Read the model definition and answer for the solid it produces. Units are mm, in the model's axes. A direction names the side the tool comes from. Round coordinates to 2 decimals unless told otherwise and drop trailing zeros. Order: outer loops, then holes, each group sorted by start corner. A loop starts at its lowest first (then second) coordinate and runs counter-clockwise, first axis right, second up. Notation, with made-up numbers: (19.25, 19.25) - (26.25, 19.25) arc R9 ccw to (26.25, 30.25) - close; hole circle Ø1 at (-19.75, 26). An arc over 180 degrees is marked (long way). Put each result on its own line as item: value. Start each with the question number.
Q1. Section A-A on y = 10.5 is taken. Give the vertices of the cut face in (x, z).
Q2. Find the intervals of material crossed by line 1 along Y through (x, z) = (78, 0.9); line 2 along X through (y, z) = (9, 0.65); line 3 along Y through (x, z) = (-83, 2.6), in increasing order. Write a range as from..to.
Q3. Which of the six approach directions +Z, -Z, +X, -X, +Y, -Y give full straight-line access (tool end or side, diameter ignored) to faces 4 (the face through (52.5, -21, 2)), 5 (the face through (-87, -20, 1)), 6 (the face through (0, 20, 1)), 7 (the face through (86, -20, 1))?
Q4. For a pull along X with two mould halves and no side action, classify faces 1 (the face through (89, -1, 1)), 2 (the face through (-90.5, -18, 1)), 3 (the face through (52.5, 22, 2)) as pulls with the +X half, pulls with the -X half, needs draft (parallel to the pull), parting line crosses it, or undercut.
Q5. Section C-C on y = -7 is taken. Give the vertices of the cut face in (x, z).
Q6. Each of these flat-tipped pins is pushed along its axis until it touches: pin 1 Ø0.9 at (x, z) = (-3.5, 2) entering from +Y; pin 2 Ø1.5 at (x, z) = (89, 1.5) entering from +Y; pin 3 Ø1.5 at (x, z) = (30.5, 1.5) entering from -Y. Where does it stop, or does it pass through?
Q7. Section B-B on x = 78 is taken. Give the vertices of the cut face in (y, z).
Q8. Section D-D on z = 2.05 is taken. State how many separate pieces and enclosed holes the cut face has, then the cut area to 3 significant figures.
Autodesk Inventor part; units mm, degrees
ref_plane "YZ Plane" through (0, 0, 0) normal (1, 0, 0) x (0, 1, 0)
ref_plane "XZ Plane" through (0, 0, 0) normal (0, 1, 0) x (-1, 0, 0)
ref_plane "XY Plane" through (0, 0, 0) normal (0, 0, 1) x (1, 0, 0)
sketch "Sketch1" plane through (0, 0, 0) normal (0, 0, 1) x (1, 0, 0)
  line L0 (-87.5, -20) -> (87.5, -20)
  line L1 (87.5, -20) -> (87.5, 20)
  line L2 (87.5, 20) -> (-87.5, 20)
  line L3 (-87.5, 20) -> (-87.5, -20)
  line L4 (-87.5, -20) -> (87.5, 20) construction
  line L5 (87.5, -20) -> (-87.5, 20) construction
  line L6 (-87.5, 14) -> (-90.5, 14)
  line L7 (-90.5, 14) -> (-90.5, -1)
  line L8 (-90.5, -1) -> (-87.5, -1)
  line L9 (-87.5, -1) -> (-87.5, 14)
  line L10 (-87.5, -20) -> (-90.5, -20)
  line L11 (-90.5, -20) -> (-90.5, -16)
  line L12 (-90.5, -16) -> (-87.5, -16)
  line L13 (-87.5, -16) -> (-87.5, -20)
  line L14 (0, 20) -> (0, -20) construction
  line L15 (87.5, 14) -> (90.5, 14)
  line L16 (90.5, 14) -> (90.5, -1)
  line L17 (90.5, -1) -> (87.5, -1)
  line L18 (87.5, -1) -> (87.5, 14)
  line L19 (87.5, -20) -> (90.5, -20)
  line L20 (90.5, -20) -> (90.5, -16)
  line L21 (90.5, -16) -> (87.5, -16)
  line L22 (87.5, -16) -> (87.5, -20)
  point P0 (0, 0)
  dimension "d0" = 175
  dimension "d1" = 40
  dimension "d2" = 3
  dimension "d3" = 15
  dimension "d4" = 6
  dimension "d5" = 3
  dimension "d6" = 15
extrude "Extrusion1" add sketch "Sketch1" along normal blind 3
sketch "Sketch2" plane through (0, 0, 3) normal (0, 0, 1) x (1, 0, 0)
  line L0 (-90.5, -20) -> (90.5, -20)
  line L1 (-82.5, -20) -> (-67.5, -20)
  line L2 (-67.5, -20) -> (-67.5, -23)
  line L3 (-67.5, -23) -> (-82.5, -23)
  line L4 (-82.5, -23) -> (-82.5, -20)
  line L5 (-52.5, -20) -> (-37.5, -20)
  line L6 (-37.5, -20) -> (-37.5, -23)
  line L7 (-37.5, -23) -> (-52.5, -23)
  line L8 (-52.5, -23) -> (-52.5, -20)
  line L9 (-22.5, -20) -> (-7.5, -20)
  line L10 (-7.5, -20) -> (-7.5, -23)
  line L11 (-7.5, -23) -> (-22.5, -23)
  line L12 (-22.5, -23) -> (-22.5, -20)
  line L13 (7.5, -20) -> (22.5, -20)
  line L14 (22.5, -20) -> (22.5, -23)
  line L15 (22.5, -23) -> (7.5, -23)
  line L16 (7.5, -23) -> (7.5, -20)
  line L17 (37.5, -20) -> (52.5, -20)
  line L18 (52.5, -20) -> (52.5, -23)
  line L19 (52.5, -23) -> (37.5, -23)
  line L20 (37.5, -23) -> (37.5, -20)
  line L21 (67.5, -20) -> (82.5, -20)
  line L22 (82.5, -20) -> (82.5, -23)
  line L23 (82.5, -23) -> (67.5, -23)
  line L24 (67.5, -23) -> (67.5, -20)
  line L25 (-82.5, 23) -> (-67.5, 23)
  line L26 (-67.5, 23) -> (-67.5, 20)
  line L27 (-67.5, 20) -> (-82.5, 20)
  line L28 (-82.5, 20) -> (-82.5, 23)
  line L29 (-52.5, 23) -> (-37.5, 23)
  line L30 (-37.5, 23) -> (-37.5, 20)
  line L31 (-37.5, 20) -> (-52.5, 20)
  line L32 (-52.5, 20) -> (-52.5, 23)
  line L33 (-22.5, 23) -> (-7.5, 23)
  line L34 (-7.5, 23) -> (-7.5, 20)
  line L35 (-7.5, 20) -> (-22.5, 20)
  line L36 (-22.5, 20) -> (-22.5, 23)
  line L37 (7.5, 23) -> (22.5, 23)
  line L38 (22.5, 23) -> (22.5, 20)
  line L39 (22.5, 20) -> (7.5, 20)
  line L40 (7.5, 20) -> (7.5, 23)
  line L41 (37.5, 23) -> (52.5, 23)
  line L42 (52.5, 23) -> (52.5, 20)
  line L43 (52.5, 20) -> (37.5, 20)
  line L44 (37.5, 20) -> (37.5, 23)
  line L45 (67.5, 23) -> (82.5, 23)
  line L46 (82.5, 23) -> (82.5, 20)
  line L47 (82.5, 20) -> (67.5, 20)
  line L48 (67.5, 20) -> (67.5, 23)
  line L49 (-90.5, -16) -> (-90.5, -20)
  line L50 (-87.5, -16) -> (-90.5, -16)
  point P0 (0, 0)
  point P1 (0, 0)
  dimension "d13" = 15
  dimension "d14" = 3
  dimension "d16" = 30
  dimension "d17" = 43
  dimension "d18" = 8
  dimension "d19" = 4
extrude "Extrusion2" add sketch "Sketch2" against normal blind 3
sketch "Sketch3" plane through (0, 0, 3) normal (0, 0, 1) x (1, 0, 0)
  circle A0 centre (-78, 10.5) radius 2
  circle A1 centre (78, 10.5) radius 2
  line L0 (87.5, 14) -> (87.5, 20)
  line L1 (87.5, 20) -> (82.5, 20)
  line L2 (-52.5, 20) -> (-67.5, 20)
  line L3 (-87.5, 20) -> (-87.5, 14)
  point P0 (0, 0)
  dimension "d22" = 4
  dimension "d23" = 4
  dimension "d24" = 9.5
  dimension "d25" = 9.5
  dimension "d26" = 9.5
  dimension "d27" = 9.5
extrude "Extrusion3" cut sketch "Sketch3" against normal blind 10
equation "\"BendRadius\" = Thickness"
equation "\"BendReliefWidth\" = Thickness"
equation "\"BendReliefDepth\" = 0.5 * Thickness"
equation "\"CornerReliefSize\" = 4 * Thickness"
equation "\"MinimumRemnant\" = 2 * Thickness"
equation "\"TransitionRadius\" = BendRadius"
equation "\"JacobiRadiusSize\" = BendRadius"
equation "\"GapSize\" = Thickness"
properties part number "13 achter plaat LCD"
Findings:
1. outline: (-90.5, 0) - (-80, 0) - (-80, 3) - (-90.5, 3) - close; (-76, 0) - (76, 0) - (76, 3) - (-76, 3) - close; (80, 0) - (90.5, 0) - (90.5, 3) - (80, 3) - close
2. line 1: -23..8.5, 12.5..23
2. line 2: -90.5..-79.32, -76.68..76.68, 79.32..90.5
2. line 3: -20..20
3. face 4: +Z, -Z, -Y
3. face 5: +Z, -Z, -X, -Y
3. face 6: +Z, -Z, +Y
3. face 7: +Z, -Z, +X, -Y
4. face 1: needs draft
4. face 2: pulls with the -X half
4. face 3: undercut
5. outline: (-87.5, 0) - (87.5, 0) - (87.5, 3) - (-87.5, 3) - close
6. pin 1: y = 20
6. pin 2: y = 14
6. pin 3: y = -20
7. outline: (-23, 0) - (8.5, 0) - (8.5, 3) - (-23, 3) - close; (12.5, 0) - (23, 0) - (23, 3) - (12.5, 3) - close
8. separate pieces: 1
8. enclosed holes: 2
8. area: 7,630 mm2
